Geometry: final body of the model. Coordinates: model frame, mm. Face numbers are marked on the shaded views. A direction names the side the tool comes from. Round coordinates to 2 decimals unless told otherwise and drop trailing zeros. Loops run counter-clockwise (first coordinate to the right, second up) from the corner with the lowest first, then second, coordinate; pieces in that order, holes last. Notation, with made-up numbers: M 57.5,-9.5 L 92.5,-9.5 A14 cw 92.5,13.5 Z; hole C 43,75.25 d8. An arc over 180 degrees is marked long. Return JSON: item names as keys, results as strings.
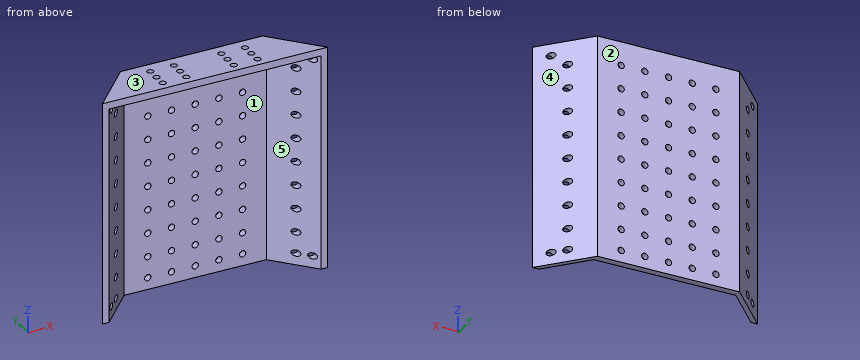
from build123d import *

# Parameters (mm, degrees)
CROQUIS2_W                     = 60
CROQUIS2_H                     = 19
SALIENTE_EXTRUIR1_DEPTH        = 94
CORTAR_EXTRUIR1_DEPTH          = 91
TALADRO_DE_MARGEN_PARA_M2_51_D = 2.7
TALADRO_DE_MARGEN_PARA_M2_52_D = 2.7


with BuildPart() as part:
    # Croquis2 → Saliente-Extruir1 (new body)
    with BuildSketch(Plane.XY):
        with Locations((0, 9.5)):
            Rectangle(CROQUIS2_W, CROQUIS2_H)
        Polygon((-30, 0), (-30, 19), (-47.5, 0), align=None)
        Polygon((47.5, 0), (30, 0), (30, 19), align=None)
    extrude(amount=SALIENTE_EXTRUIR1_DEPTH)

    # Croquis3 → Cortar-Extruir1 (cut)
    with BuildSketch(Plane(origin=(0, 0, 0), x_dir=(-1, 0, 0), z_dir=(0, 0, -1))):
        Polygon((-30, 16), (-44.736842105, 0), (44.736842105, 0), (30, 16), align=None)
    extrude(amount=-CORTAR_EXTRUIR1_DEPTH, mode=Mode.SUBTRACT)

    # Taladro de margen para M2.51 (through all)
    with Locations(Plane(origin=(0, 19, 0), x_dir=(1, 0, 0), z_dir=(0, 1, 0))):
        with Locations((-42.5, -5), (42.5, -5), (42.5, -89), (-42.5, -89), (-38, -5), (-38, -14), (-38, -24), (-38, -34), (-38, -44), (-38, -54), (-38, -64), (-38, -74), (-38, -84), (-20, -5), (-20, -14), (-20, -24), (-20, -34), (-20, -44), (-20, -54), (-20, -64), (-20, -74), (-20, -84), (0, -5), (0, -14), (0, -24), (0, -34), (0, -44), (0, -54), (0, -64), (0, -74), (0, -84), (20, -5), (20, -14), (20, -24), (20, -34), (20, -44), (20, -54), (20, -64), (20, -74), (20, -84), (38, -5), (38, -14), (38, -24), (38, -34), (38, -44), (38, -54), (38, -64), (38, -74), (38, -84), (-10, -5), (-10, -14), (-10, -24), (-10, -34), (-10, -44), (-10, -54), (-10, -64), (-10, -74), (-10, -84), (10, -5), (10, -14), (10, -24), (10, -34), (10, -44), (10, -54), (10, -64), (10, -74), (10, -84)):
            Hole(TALADRO_DE_MARGEN_PARA_M2_51_D / 2)

    # Taladro de margen para M2.52 (through all)
    with Locations(Plane(origin=(-20, 14, 94), x_dir=(1, 0, 0), z_dir=(0, 0, 1))):
        with Locations((0, 0), (0, -5), (0, -10.037142857), (10, -10.037142857), (10, -5), (10, 0), (30, -10.037142857), (30, -5), (30, 0), (40, 0), (40, -5), (40, -10.037142857)):
            Hole(TALADRO_DE_MARGEN_PARA_M2_52_D / 2)


solid = part.part
Q1. Section query A-A (y = 14). Output: boundary loops of the cut face in (x, z).
Determined:
{"outline": "M -34.61,0 L -31.84,0 L -31.84,91 L -21.35,91 L -21.35,94 L -34.61,94 Z; M -18.65,91 L -11.35,91 L -11.35,94 L -18.65,94 Z; M -8.65,91 L 8.65,91 L 8.65,94 L -8.65,94 Z; M 11.35,91 L 18.65,91 L 18.65,94 L 11.35,94 Z; M 21.35,91 L 31.84,91 L 31.84,0 L 34.61,0 L 34.61,94 L 21.35,94 Z"}
Q2. Pull-direction query (X, two-part tool) for the marked faces 3, 4 and 5; classes: pulls with the +X half, pulls with the -X half, needs draft (parallel to the pull), parting line crosses it, or undercut.
Determined:
{"face 3": "needs draft", "face 4": "pulls with the +X half", "face 5": "undercut"}
Q3. Section query D-D (z = 89). Output: boundary loops of the cut face in (x, y), plus the area to 3 significant figures.
Determined:
{"outline": "M -47.5,0 L -44.74,0 L -43.85,0.96 L -43.85,3.96 Z; M -41.15,3.89 L -30,16 L 30,16 L 41.15,3.89 L 41.15,6.89 L 30,19 L -30,19 L -41.15,6.89 Z; M 43.85,0.96 L 44.74,0 L 47.5,0 L 43.85,3.96 Z", "area": "261 mm^2"}
Q4. Reachability of the marked faces 1 and 2 from +Z, -Z, +X, -X, +Y, -Y: full face, straight path, thin tool, end or side. Return the list, or none.
Determined:
{"face 1": "-Z, -Y", "face 2": "+Z, -Z, +X, -X, +Y"}
Q5. Section query B-B (z = 7.5). Output: boundary loops of the cut face in (x, y), plus the area to 3 significant figures.
Determined:
{"outline": "M -47.5,0 L -44.74,0 L -30,16 L 30,16 L 44.74,0 L 47.5,0 L 30,19 L -30,19 Z", "area": "277 mm^2"}
Q6. Material intervals for L1, parallel to X at y = 17.9, z = 74; L2, parallel to X at y = 17.65, z = 84; L3, parallel to Y at x = 13, z = 73.5, sorted ascending.
Determined:
{"L1": "x = -31.01 to -21.35, -18.65 to -11.35, -8.65 to -1.35, 1.35 to 8.65, 11.35 to 18.65, 21.35 to 31.01", "L2": "x = -31.24 to -21.35, -18.65 to -11.35, -8.65 to -1.35, 1.35 to 8.65, 11.35 to 18.65, 21.35 to 31.24", "L3": "y = 16 to 19"}
Q7. Section query C-C (x = -20). State how many separate pieces and enclosed holes the cut face has, plus the area to 3 significant figures.
Determined:
{"separate pieces": "13", "enclosed holes": "0", "area": "233 mm^2"}
Q8. Pin query (flat end, axial travel): pin 1 (4 mm diameter, centred on y = 15, z = 15.5, fed in from +X); pin 2 (3 mm diameter, centred on x = 38, z = 5, fed in from +Y); pin 3 (1.6 mm diameter, centred on x = 0, z = 84, fed in from -Y); pin 4 (3.5 mm diameter, centred on x = 10, z = 74, fed in from -Y). Return the tip coordinate at first contact, or that it passes through.
Determined:
{"pin 1": "stops at x = 35.53", "pin 2": "stops at y = 11.94", "pin 3": "passes through", "pin 4": "stops at y = 16"}
